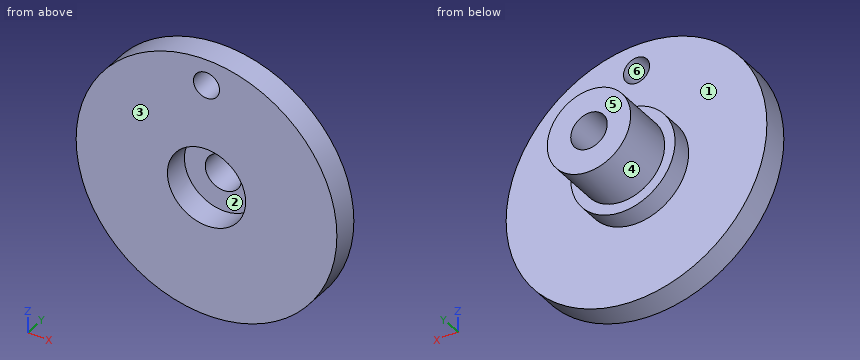
Autodesk Inventor part; units mm, degrees
ref_plane "YZ Plane" through (0, 0, 0) normal (1, 0, 0) x (0, 1, 0)
ref_plane "XZ Plane" through (0, 0, 0) normal (0, 1, 0) x (-1, 0, 0)
ref_plane "XY Plane" through (0, 0, 0) normal (0, 0, 1) x (1, 0, 0)
sketch "Sketch1" plane through (0, 0, 0) normal (0, 1, 0) x (-1, 0, 0)
  circle A0 centre (0, 0) radius 25
  dimension "d0" = 50
extrude "Extrusion1" add sketch "Sketch1" along normal blind 5
sketch "Sketch2" plane through (0, 5, 0) normal (0, 1, 0) x (1, 0, 0)
  circle A0 centre (0, 0) radius 7.5
  dimension "d3" = 15
extrude "Extrusion2" cut sketch "Sketch2" against normal through all
sketch "Sketch4" plane through (0, 5, 0) normal (0, 1, 0) x (1, 0, 0)
  circle A0 centre (0, 0) radius 20 construction
  circle A1 centre (0, -20) radius 2.5
  dimension "d8" = 40
  dimension "d9" = 5
extrude "Extrusion3" cut sketch "Sketch4" against normal through all
sketch "Sketch5" plane through (0, 0, 0) normal (0, -1, 0) x (1, 0, 0)
  line L0 (0, 0) -> (0, 34) construction
  circle A0 centre (0, 20) radius 2.5 construction
  circle A1 centre (0, 0) radius 7.5 construction
  circle A2 centre (0, 0) radius 25 construction
sketch "Sketch6" plane through (0, 5, 0) normal (0, 1, 0) x (1, 0, 0)
  circle A0 centre (0, 0) radius 10
  dimension "d12" = 20
extrude "Extrusion4" add sketch "Sketch6" along normal blind 4
sketch "Sketch7" plane through (0, 9, 0) normal (0, 1, 0) x (1, 0, 0)
  circle A0 centre (0, 0) radius 8
  dimension "d15" = 16
extrude "Extrusion5" add sketch "Sketch7" along normal blind 10
sketch "Sketch8" plane through (0, 19, 0) normal (0, 1, 0) x (1, 0, 0)
  circle A0 centre (0, 0) radius 3.5
  dimension "d18" = 7
extrude "Extrusion6" cut sketch "Sketch8" against normal through all
properties part number "sprzeglo_01"
Read the model definition and answer for the solid it produces. Units are mm, in the model's axes. Face numbers are marked on the shaded views. A direction names the side the tool comes from. Coordinates: 2 decimals unless noted, no trailing zeros. Write each loop counter-clockwise with the first axis right and the second up, starting at its lowest first coordinate (ties: lowest second). Pieces come first, ordered by that corner, then holes. Notation, with made-up numbers: (0, -15.5) - (23, -15.5) arc R17 ccw to (23, 5.5) - close; hole circle Ø9 at (85.25, 73.5). An arc over 180 degrees is marked (long way). One line per question, with ' | ' between items.
Q1. Find section B-B, the plane x = 0. Write down the section's boundary in (y, z), plus the area to 3 significant figures.
Result set:
outline: (0, -25) - (5, -25) - (5, -10) - (9, -10) - (9, -8) - (19, -8) - (19, -3.5) - (5, -3.5) - (5, -7.5) - (0, -7.5) - close; (0, 7.5) - (5, 7.5) - (5, 3.5) - (19, 3.5) - (19, 8) - (9, 8) - (9, 10) - (5, 10) - (5, 17.5) - (0, 17.5) - close; (0, 22.5) - (5, 22.5) - (5, 25) - (0, 25) - close | area: 292 mm^2
Q2. Determine the mould class of the marked faces 4, 5 and 6 for opening direction X: +X half, -X half, draft (parallel to the pull), parting line (faces both ways), or undercut.
Result set:
face 4: parting line | face 5: draft | face 6: undercut
Q3. Find section C-C, the plane y = 13. Write down the section's boundary in (x, z).
Result set:
outline: circle Ø16 at (0, 0); hole circle Ø7 at (0, 0)
Q4. Each of these flat-tipped pins is pushed along its axis until it touches: P1, Ø8, axis at y = 6.5, z = -9, coming from the +X side; P2, Ø8, axis at x = 8, z = -14, coming from the -Y side; P3, Ø11, axis at x = 0, z = 0, coming from the -Y side; P4, Ø1.5, axis at x = 18.5, z = -10.5, coming from the +Y side. Where does it stop, or does it pass through?
Result set:
P1: x = 24.43 | P2: y = 0 | P3: y = 5 | P4: y = 5
Q5. For the marked faces 1, 2 and 3, determine the directions among +Z, -Z, +X, -X, +Y, -Y from which every point of the face is accessible in a straight line to the end or side of a thin tool.
Result set:
face 1: +Y | face 2: -Y | face 3: +Z, -Z, +X, -X, -Y
Q6. Find section A-A, the plane z = 0. Write down the section's boundary in (x, y).
Result set:
outline: (-25, 0) - (-7.5, 0) - (-7.5, 5) - (-3.5, 5) - (-3.5, 19) - (-8, 19) - (-8, 9) - (-10, 9) - (-10, 5) - (-25, 5) - close; (3.5, 5) - (7.5, 5) - (7.5, 0) - (25, 0) - (25, 5) - (10, 5) - (10, 9) - (8, 9) - (8, 19) - (3.5, 19) - close
Q7. Find section D-D, the plane z = 20. Write down the section's boundary in (x, y).
Result set:
outline: (-15, 0) - (-2.5, 0) - (-2.5, 5) - (-15, 5) - close; (2.5, 0) - (15, 0) - (15, 5) - (2.5, 5) - close
Q8. Consider L1, parallel to Z at x = 0, y = 1.6; L2, parallel to Z at x = 0, y = 13.25; L3, parallel to Z at x = -1, y = 4. Determine where each line is inside the solid, lowest interval first. Write a range as [from, to].
Result set:
L1: [-25, -7.5], [7.5, 17.5], [22.5, 25] | L2: [-8, -3.5], [3.5, 8] | L3: [-24.98, -7.43], [7.43, 17.71], [22.29, 24.98]
